The listing builds one solid part. Answer for the finished solid, in the listing's coordinates (mm). Face numbers are marked on the shaded views. A direction names the side the tool comes from. Round coordinates to 2 decimals unless told otherwise and drop trailing zeros. Write each loop counter-clockwise with the first axis right and the second up, starting at its lowest first coordinate (ties: lowest second). Pieces come first, ordered by that corner, then holes. Notation, with made-up numbers: (-19.5, 55) - (-15.5, 55) arc R19 ccw to (-15.5, 63) - close; hole circle Ø7 at (63.5, -7). An arc over 180 degrees is marked (long way). Use a Markdown table: item, result. Add a question column.
1) A cutting plane is placed at B-B (x = 0). Give the vertices of the cut face in (y, z).
2) Each of these flat-tipped pins is pushed along its axis until it touches: P1, Ø11, axis at x = -7, y = 0.5, coming from the +Z side; P2, Ø6.5, axis at x = 0, y = 0, coming from the -Z side; P3, Ø2.5, axis at y = -12, z = 4.5, coming from the -X side; P4, Ø4, axis at y = -14, z = 5.5, coming from the +X side. Where does it stop, or does it pass through?
3) A cutting plane is placed at C-C (z = 2.5). Give the vertices of the cut face in (x, y).
4) A tool of negligible diameter and unlimited length cuts with its end or side. For the marked faces 5, 6, 7 and 8, from which of +Z, -Z, +X, -X, +Y, -Y can it reach the whole face along a straight path? Write none if from no direction.
5) A cutting plane is placed at A-A (y = 8.5). Give the vertices of the cut face in (x, z).
6) Determine the mould class of the marked faces 1, 2, 3 and 4 for opening direction Y: +Y half, -Y half, draft (parallel to the pull), parting line (faces both ways), or undercut.
7) Find the intervals of material crossed by probe 1 along X at (y, z) = (-15, 4.75); probe 2 along Z at (x, y) = (0, -9); probe 3 along Y at (x, z) = (-2.75, 4), in increasing order. Write a range as from..to.
8) A cutting plane is placed at D-D (y = 0). Give the vertices of the cut face in (x, z).
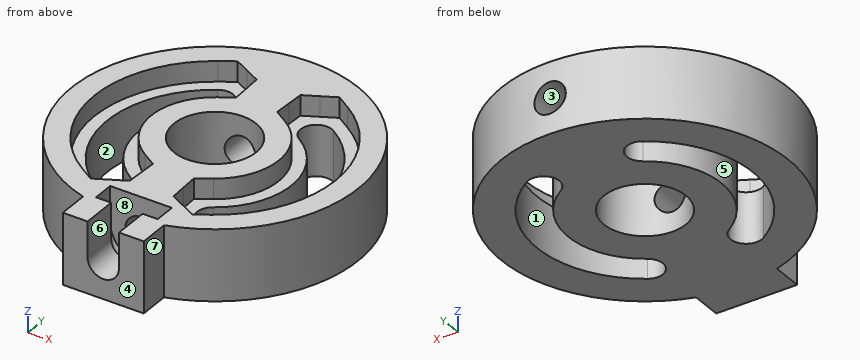
```python
from build123d import *

# Parameters (mm, degrees)
SKETCH_R        = 4.05
EXTRUDE_DEPTH   = 7
SKETCH001_R     = 1.55
POCKET_DEPTH    = 30.723859
POCKET001_DEPTH = 3.5
POCKET002_DEPTH = 2.1
POCKET003_DEPTH = 2


with BuildPart() as part:
    # Sketch → Extrude (new body)
    with BuildSketch(Plane.XY):
        with BuildLine():
            ThreePointArc((4, -13.572859), (0, 14.15), (-4, -13.572859))
            Line((-4, -13.572859), (-4, -16.572859))
            Line((-4, -16.572859), (4, -16.572859))
            Line((4, -16.572859), (4, -13.572859))
        make_face()
        Circle(SKETCH_R, mode=Mode.SUBTRACT)
        with BuildLine():
            ThreePointArc((-4.056612, 6.367605), (-7.55, 0), (-4.056612, -6.367605))
            ThreePointArc((-5.722241, -8.982119), (-3.58217, -8.507677), (-4.056612, -6.367605))
            ThreePointArc((-5.722241, 8.982119), (-10.65, 0), (-5.722241, -8.982119))
            ThreePointArc((-4.056612, 6.367605), (-3.58217, 8.507677), (-5.722241, 8.982119))
        make_face(mode=Mode.SUBTRACT)
        with BuildLine():
            ThreePointArc((4.056612, -6.367605), (7.55, 0), (4.056612, 6.367605))
            ThreePointArc((5.722241, 8.982119), (3.58217, 8.507677), (4.056612, 6.367605))
            ThreePointArc((5.722241, -8.982119), (10.65, 0), (5.722241, 8.982119))
            ThreePointArc((4.056612, -6.367605), (3.58217, -8.507677), (5.722241, -8.982119))
        make_face(mode=Mode.SUBTRACT)
    extrude(amount=EXTRUDE_DEPTH)

    # Sketch001 → Pocket (cut, through all)
    with BuildSketch(Plane.XZ.offset(16.572859)):
        with Locations((0, 3.5)):
            Circle(SKETCH001_R)
    extrude(amount=-POCKET_DEPTH, mode=Mode.SUBTRACT)

    # Sketch002 → Pocket001 (cut)
    with BuildSketch(Plane.XY.offset(7)):
        Polygon((-3.049999, -10.972859), (-3.049999, -13.072859), (-1.549999, -13.072859), (-1.549999, -16.572859), (1.550001, -16.572859), (1.550001, -13.072859), (3.050001, -13.072859), (3.050001, -10.972859), align=None)
    extrude(amount=-POCKET001_DEPTH, mode=Mode.SUBTRACT)

    # Sketch003 → Pocket002 (cut)
    with BuildSketch(Plane.XZ.offset(10.972859)):
        with BuildLine():
            ThreePointArc((-3.050001, 3.5), (0, 0.449999), (3.050001, 3.5))
            Line((-3.050001, 3.5), (3.050001, 3.5))
        make_face()
    extrude(amount=POCKET002_DEPTH, mode=Mode.SUBTRACT)

    # Sketch004 → Pocket003 (cut)
    with BuildSketch(Plane.XY.offset(7)):
        with BuildLine():
            ThreePointArc((-3.384988, 5.313366), (-6.3, 0), (-3.384988, -5.313366))
            Line((-3.384988, -5.313366), (-2.021577, -6.181954))
            Line((-2.021577, -6.181954), (-2.092091, -7.796996))
            Line((-2.092091, -7.796996), (-2.162606, -9.412039))
            Line((-2.162606, -9.412039), (-3.59653, -10.158493))
            Line((-3.59653, -10.158493), (-5.030455, -10.904946))
            Line((-5.030455, -10.904946), (-6.393865, -10.036358))
            ThreePointArc((-6.393865, 10.036358), (-11.9, 0), (-6.393865, -10.036358))
            Line((-6.393865, 10.036358), (-5.030455, 10.904946))
            Line((-5.030455, 10.904946), (-3.59653, 10.158492))
            Line((-3.59653, 10.158492), (-2.162606, 9.412039))
            Line((-2.162606, 9.412039), (-2.092091, 7.796997))
            Line((-2.092091, 7.796997), (-2.021577, 6.181954))
            Line((-2.021577, 6.181954), (-3.384988, 5.313366))
        make_face()
        with BuildLine():
            ThreePointArc((3.384988, -5.313366), (6.3, 0), (3.384988, 5.313366))
            Line((3.384988, 5.313366), (2.021577, 6.181954))
            Line((2.021577, 6.181954), (2.092091, 7.796996))
            Line((2.092091, 7.796996), (2.162606, 9.412039))
            Line((2.162606, 9.412039), (3.59653, 10.158493))
            Line((3.59653, 10.158493), (5.030455, 10.904946))
            Line((5.030455, 10.904946), (6.393865, 10.036358))
            ThreePointArc((6.393865, -10.036358), (11.9, 0), (6.393865, 10.036358))
            Line((5.030457, -10.904952), (6.393865, -10.036358))
            Line((3.596533, -10.158494), (5.030457, -10.904952))
            Line((2.16261, -9.412036), (3.596533, -10.158494))
            Line((2.092091, -7.796993), (2.16261, -9.412036))
            Line((2.021573, -6.18195), (2.092091, -7.796993))
            Line((3.384988, -5.313366), (2.021573, -6.18195))
        make_face()
    extrude(amount=-POCKET003_DEPTH, mode=Mode.SUBTRACT)


solid = part.part
```
Entries:
| question | item | result |
|---|---|---|
| 1 | outline | (-16.57, 0) - (-4.05, 0) - (-4.05, 1.95) - (-10.97, 1.95) - (-10.97, 0.45) - (-13.07, 0.45) - (-13.07, 1.95) - (-16.57, 1.95) - close; (-10.97, 5.05) - (-4.05, 5.05) - (-4.05, 7) - (-10.97, 7) - close; (4.05, 0) - (14.15, 0) - (14.15, 1.95) - (4.05, 1.95) - close; (4.05, 5.05) - (14.15, 5.05) - (14.15, 7) - (4.05, 7) - close |
| 2 | P1 | stops at z = 7 |
| 2 | P2 | passes through |
| 2 | P3 | stops at x = -9.2 |
| 2 | P4 | stops at x = 7.5 |
| 3 | outline | (-4, -16.57) - (-1.18, -16.57) - (-1.18, -13.07) - (-2.88, -13.07) - (-2.88, -10.97) - (-1.18, -10.97) - (-1.18, -3.87) arc R4.05 cw to (-1.18, 3.87) - (-1.18, 14.1) arc R14.15 ccw to (-4, -13.57) - close; (1.18, -16.57) - (4, -16.57) - (4, -13.57) arc R14.15 ccw to (1.18, 14.1) - (1.18, 3.87) arc R4.05 cw to (1.18, -3.87) - (1.18, -10.97) - (2.88, -10.97) - (2.88, -13.07) - (1.18, -13.07) - close; hole (-5.72, -8.98) arc R1.55 ccw to (-4.06, -6.37) arc R7.55 cw to (-4.06, 6.37) arc R1.55 ccw to (-5.72, 8.98) arc R10.65 ccw to start; hole (4.06, -6.37) arc R1.55 ccw to (5.72, -8.98) arc R10.65 ccw to (5.72, 8.98) arc R1.55 ccw to (4.06, 6.37) arc R7.55 cw to start |
| 4 | face 5 | +Z, -Z |
| 4 | face 6 | +Z, -Y |
| 4 | face 7 | +Z, -Z, +X, -Y |
| 4 | face 8 | +Z |
| 5 | outline | (-11.31, 0) - (-6.42, 0) - (-6.42, 5) - (-8.33, 5) - (-8.33, 7) - (-11.31, 7) - close; (-3.58, 0) - (3.58, 0) - (3.58, 5) - (2.12, 5) - (2.12, 7) - (-2.12, 7) - (-2.12, 5) - (-3.58, 5) - close; (6.42, 0) - (11.31, 0) - (11.31, 7) - (8.33, 7) - (8.33, 5) - (6.42, 5) - close; hole circle Ø3.1 at (0, 3.5) |
| 6 | face 1 | undercut |
| 6 | face 2 | undercut |
| 6 | face 3 | draft |
| 6 | face 4 | -Y half |
| 7 | probe 1 | x = -4..-1.55, 1.55..4 |
| 7 | probe 2 | z = 0..1.95, 5.05..7 |
| 7 | probe 3 | y = -16.57..-13.07, -10.97..-2.97, 2.97..13.88 |
| 8 | outline | (-14.15, 0) - (-10.65, 0) - (-10.65, 5) - (-11.9, 5) - (-11.9, 7) - (-14.15, 7) - close; (-7.55, 0) - (-4.05, 0) - (-4.05, 7) - (-6.3, 7) - (-6.3, 5) - (-7.55, 5) - close; (4.05, 0) - (7.55, 0) - (7.55, 5) - (6.3, 5) - (6.3, 7) - (4.05, 7) - close; (10.65, 0) - (14.15, 0) - (14.15, 7) - (11.9, 7) - (11.9, 5) - (10.65, 5) - close |
